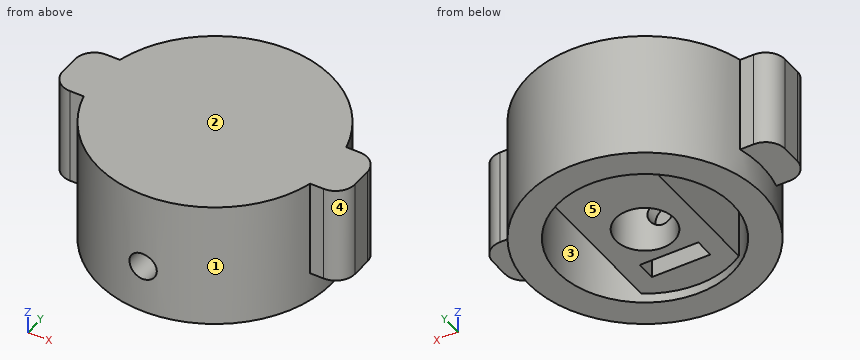
```python
from build123d import *

# Parameters (mm, degrees)
BOX003_W          = 5
BOX003_H          = 6
BOX003_DEPTH      = 10
FILLET_R          = 2
BOX002_W          = 5
BOX002_H          = 6
BOX002_DEPTH      = 10
FILLET001_R       = 2
CYLINDER005_R     = 1.4
CYLINDER005_DEPTH = 11
CYLINDER004_R     = 9
CYLINDER004_DEPTH = 1
CYLINDER003_R     = 1.4
CYLINDER003_DEPTH = 11
BOX001_W          = 6
BOX001_H          = 2
BOX001_DEPTH      = 12
CYLINDER002_R     = 3
CYLINDER002_DEPTH = 12
BOX_W             = 10
BOX_H             = 20
BOX_DEPTH         = 12
CYLINDER001_R     = 9
CYLINDER001_DEPTH = 11
CYLINDER_R        = 12
CYLINDER_DEPTH    = 13


with BuildPart() as fillet_body:
    # Box003 → Box003 (new body)
    with BuildSketch(Plane(origin=(-15, -3, 3), x_dir=(1, 0, 0), z_dir=(0, 0, 1))):
        with Locations((2.5, 3)):
            Rectangle(BOX003_W, BOX003_H)
    extrude(amount=BOX003_DEPTH)

    # Fillet
    fillet_edges = [fillet_body.edges().sort_by_distance(p)[0] for p in [
        (-15, -3, 8),
        (-15, 3, 8),
    ]]
    fillet(fillet_edges, radius=FILLET_R)


with BuildPart() as fillet001:
    # Box002 → Box002 (new body)
    with BuildSketch(Plane(origin=(10, -3, 3), x_dir=(1, 0, 0), z_dir=(0, 0, 1))):
        with Locations((2.5, 3)):
            Rectangle(BOX002_W, BOX002_H)
    extrude(amount=BOX002_DEPTH)

    # Fillet001
    fillet001_edges = [fillet001.edges().sort_by_distance(p)[0] for p in [
        (15, -3, 8),
        (15, 3, 8),
    ]]
    fillet(fillet001_edges, radius=FILLET001_R)


with BuildPart() as cylinder005:
    # Cylinder005 → Cylinder005 (new body)
    with BuildSketch(Plane(origin=(0, -2, 5), x_dir=(1, 0, 0), z_dir=(0, -1, 0))):
        Circle(CYLINDER005_R)
    extrude(amount=CYLINDER005_DEPTH)


with BuildPart() as cylinder004:
    # Cylinder004 → Cylinder004 (new body)
    with BuildSketch(Plane.XY):
        Circle(CYLINDER004_R)
    extrude(amount=CYLINDER004_DEPTH)


with BuildPart() as cylinder003:
    # Cylinder003 → Cylinder003 (new body)
    with BuildSketch(Plane(origin=(0, -2, 5), x_dir=(1, 0, 0), z_dir=(0, -1, 0))):
        Circle(CYLINDER003_R)
    extrude(amount=CYLINDER003_DEPTH)


with BuildPart() as cube001:
    # Box001 → Box001 (new body)
    with BuildSketch(Plane(origin=(-3, -6, 0), x_dir=(1, 0, 0), z_dir=(0, 0, 1))):
        with Locations((3, 1)):
            Rectangle(BOX001_W, BOX001_H)
    extrude(amount=BOX001_DEPTH)


with BuildPart() as cylinder002:
    # Cylinder002 → Cylinder002 (new body)
    with BuildSketch(Plane.XY):
        Circle(CYLINDER002_R)
    extrude(amount=CYLINDER002_DEPTH)


with BuildPart() as cut003:
    # Box → Box (new body)
    with BuildSketch(Plane(origin=(-5, -10, 0), x_dir=(1, 0, 0), z_dir=(0, 0, 1))):
        with Locations((5, 10)):
            Rectangle(BOX_W, BOX_H)
    extrude(amount=BOX_DEPTH)

    # Cut001: cut Cylinder002
    add(cylinder002.part, mode=Mode.SUBTRACT)

    # Cut002: cut Cube001
    add(cube001.part, mode=Mode.SUBTRACT)

    # Cut003: cut Cylinder003
    add(cylinder003.part, mode=Mode.SUBTRACT)


with BuildPart() as cylinder001:
    # Cylinder001 → Cylinder001 (new body)
    with BuildSketch(Plane.XY):
        Circle(CYLINDER001_R)
    extrude(amount=CYLINDER001_DEPTH)


with BuildPart() as fusion001:
    # Cylinder → Cylinder (new body)
    with BuildSketch(Plane.XY):
        Circle(CYLINDER_R)
    extrude(amount=CYLINDER_DEPTH)

    # Cut: cut Cylinder001
    add(cylinder001.part, mode=Mode.SUBTRACT)

    # Fusion: union Cut003
    add(cut003.part)

    # Cut004: cut Cylinder004
    add(cylinder004.part, mode=Mode.SUBTRACT)

    # Cut005: cut Cylinder005
    add(cylinder005.part, mode=Mode.SUBTRACT)

    # Fusion001: union Fillet body, Fillet001
    add(fillet_body.part)
    add(fillet001.part)


solid = fusion001.part
```
The model under review builds one solid part; all positions refer to its coordinate system, in mm. Face numbers are marked on the shaded views. A direction names the side the tool comes from. Round coordinates to 2 decimals unless told otherwise and drop trailing zeros. Loops run counter-clockwise (first coordinate to the right, second up) from the corner with the lowest first, then second, coordinate; pieces in that order, holes last.
Item 1: Take a section at C-C (y = 0). Write out the cut boundary in (x, z).
Determined:
outline: (-15, 3) - (-12, 3) - (-12, 0) - (-9, 0) - (-9, 11) - (-5, 11) - (-5, 1) - (-3, 1) - (-3, 11) - (3, 11) - (3, 1) - (5, 1) - (5, 11) - (9, 11) - (9, 0) - (12, 0) - (12, 3) - (15, 3) - (15, 13) - (-15, 13) - close
Item 2: Clearance check with flat-ended pins moving along their axes: pin 1 Ø4.5 at (x, y) = (-6, 0) entering from -Z; pin 2 Ø1.7 at (x, y) = (14, 1) entering from -Z; pin 3 Ø1.6 at (x, y) = (-1, -5) entering from -Z. State where each tip first meets the part, or that it passes through.
Determined:
pin 1: stops at z = 1
pin 2: stops at z = 3
pin 3: stops at z = 11
Item 3: For line 1 (X direction, y = 0, z = 3.25); line 2 (Y direction, x = 0, z = 7.25); line 3 (Z direction, x = 0, y = -7.85), list the stretches that pass through material, from the lowest coordinate up.
Determined:
line 1: x = -15 to -9, -5 to -3, 3 to 5, 9 to 15
line 2: y = -12 to -6, -4 to -3, 3 to 12
line 3: z = 1 to 3.6, 6.4 to 13
Item 4: Take a section at B-B (z = 10.5). Write out the cut boundary in (x, y).
Determined:
outline: (-15, -1) arc R2 ccw to (-13, -3) - (-11.62, -3) arc R12 ccw to (11.62, -3) - (13, -3) arc R2 ccw to (15, -1) - (15, 1) arc R2 ccw to (13, 3) - (11.62, 3) arc R12 ccw to (-11.62, 3) - (-13, 3) arc R2 ccw to (-15, 1) - close; hole (-5, -7.48) - (-5, 7.48) arc R9 ccw to start; hole (-3, -6) - (3, -6) - (3, -4) - (-3, -4) - close; hole circle Ø6 at (0, 0); hole (5, -7.48) arc R9 ccw to (5, 7.48) - close
Item 5: For the marked faces 4 and 5, list the 3-axis set-ups (+Z, -Z, +X, -X, +Y, -Y) from which the entire face can be reached by the end or side of a thin tool; tool diameter is ignored.
Determined:
face 4: +Z, -Z, +X, -Y
face 5: -Z
Item 6: Mouldability with a two-part tool opening along Y and no side actions: class the marked faces 1, 2 and 3 as released by +Y, released by -Y, zero draft, split by the parting line, or undercut.
Determined:
face 1: split by the parting line
face 2: zero draft
face 3: undercut
Item 7: Take a section at A-A (x = 0). Write out the cut boundary in (y, z).
Determined:
outline: (-12, 0) - (-9, 0) - (-9, 1) - (-6, 1) - (-6, 3.6) - (-12, 3.6) - close; (-12, 6.4) - (-6, 6.4) - (-6, 11) - (-4, 11) - (-4, 6.4) - (-3, 6.4) - (-3, 11) - (3, 11) - (3, 1) - (9, 1) - (9, 0) - (12, 0) - (12, 13) - (-12, 13) - close; (-4, 1) - (-3, 1) - (-3, 3.6) - (-4, 3.6) - close
Item 8: Take a section at D-D (y = -6.5). Write out the cut boundary in (x, z), then the cut area to 3 significant figures.
Determined:
outline: (-10.09, 0) - (-6.22, 0) - (-6.22, 11) - (-5, 11) - (-5, 1) - (5, 1) - (5, 11) - (6.22, 11) - (6.22, 0) - (10.09, 0) - (10.09, 13) - (-10.09, 13) - close; hole circle Ø2.8 at (0, 5)
area: 219 mm2
